from build123d import *

# Parameters (mm, degrees)
SKETCH046_R     = 1.5
PAD026_DEPTH    = 30
POCKET016_DEPTH = 19
POCKET017_DEPTH = 50
PAD027_DEPTH    = 3
PAD028_DEPTH    = 10
SKETCH054_W     = 30
SKETCH054_H     = 5.5
POCKET020_DEPTH = 9


with BuildPart() as part:
    # Sketch046 → Pad026 (new body)
    with BuildSketch(Plane.XY):
        with BuildLine():
            Line((-21.439893, 1.606546), (-18, 1))
            Line((-18, 1), (-18, 0))
            Line((-18, 0), (-20, 0))
            Line((-20, 0), (-20, -2))
            Line((-20, -2), (-18, -2))
            Line((-18, -2), (-18, -3))
            Line((-19.218253, -3.302841), (-18, -3))
            ThreePointArc((-19.218253, -3.302841), (-18.4595, -6.284654), (-17.241169, -9.11))
            Line((17.241169, -9.11), (-17.241169, -9.11))
            ThreePointArc((17.241169, -9.11), (18.417093, -6.407863), (19.172397, -3.559379))
            Line((19.172397, -3.559379), (16, -3))
            Line((16, -3), (16, -2))
            Line((16, -2), (18, -2))
            Line((18, -2), (18, 0))
            Line((18, 0), (16, 0))
            Line((16, 0), (16, 1))
            Line((16, 1), (21.411013, 1.954108))
            ThreePointArc((13, -17.124544), (19.673032, -8.673051), (21.411013, 1.954108))
            Line((13, -17.124544), (10, -17.124544))
            Line((10, -17.124544), (10, -10.124544))
            Line((10, -10.124544), (-10, -10.124544))
            Line((-10, -10.124544), (-10, -17.124544))
            Line((-10, -17.124544), (-13, -17.124544))
            ThreePointArc((-21.439893, 1.606546), (-19.60204, -8.832328), (-13, -17.124544))
        make_face()
        with Locations((-12.5, -15)):
            Circle(SKETCH046_R, mode=Mode.SUBTRACT)
        with Locations((12.5, -15)):
            Circle(SKETCH046_R, mode=Mode.SUBTRACT)
    extrude(amount=PAD026_DEPTH)

    # Sketch047 (on Face28 of Pad026) → Pocket016 (cut)
    with BuildSketch(Plane.XY.offset(30)):
        with BuildLine():
            ThreePointArc((-18.966908, -10.124544), (-16.362176, -13.947372), (-13, -17.124544))
            Line((-13, -17.124544), (13, -17.124544))
            ThreePointArc((13, -17.124544), (16.362176, -13.947372), (18.966908, -10.124544))
            Line((-18.966908, -10.124544), (18.966908, -10.124544))
        make_face()
    extrude(amount=-POCKET016_DEPTH, mode=Mode.SUBTRACT)

    # Sketch049 (on Face5 of Pocket016) → Pocket017 (cut)
    with BuildSketch(Plane.XY.offset(30)):
        with BuildLine():
            ThreePointArc((19.172397, -3.559379), (0, 19.5), (-19.172397, -3.559379))
            Line((19.172397, -3.559379), (-19.172397, -3.559379))
        make_face()
    extrude(amount=-POCKET017_DEPTH, mode=Mode.SUBTRACT)

    # Sketch048 (on Face5 of Pocket016) → Pad027 (join)
    with BuildSketch(Plane.XY.offset(30)):
        with BuildLine():
            ThreePointArc((-21.406775, 2), (-21.077469, -4.241496), (-18.966908, -10.124544))
            Line((-7.875644, -10.124544), (-18.966908, -10.124544))
            Line((-6, -17.124544), (-7.875644, -10.124544))
            Line((6, -17.124544), (-6, -17.124544))
            Line((6, -17.124544), (7.875644, -10.124544))
            Line((7.875644, -10.124544), (18.966908, -10.124544))
            ThreePointArc((18.966908, -10.124544), (20.278323, -7.144202), (21.12463, -4))
            Line((21.12463, -4), (22.264041, -3.25))
            ThreePointArc((22.264041, -3.25), (22.220442, 3.535811), (20.155644, 10))
            Line((15.730461, 10), (20.155644, 10))
            Line((12, 2), (15.730461, 10))
            Line((12, 2), (-21.406775, 2))
        make_face()
    extrude(amount=PAD027_DEPTH)

    # Sketch053 (on Face4 of Pad027) → Pad028 (join)
    with BuildSketch(Plane(origin=(0, 0, 30), x_dir=(1, 0, 0), z_dir=(0, 0, -1))):
        with BuildLine():
            ThreePointArc((20.155644, -10), (22.220442, -3.535811), (22.264041, 3.25))
            Line((22.264041, 3.25), (19.172397, 3.559379))
            ThreePointArc((16.740669, -10), (19.193782, -3.442198), (19.172397, 3.559379))
            Line((16.740669, -10), (20.155644, -10))
        make_face()
    extrude(amount=PAD028_DEPTH)

    # Sketch054 (on Face32 of Pad028) → Pocket020 (cut)
    with BuildSketch(Plane(origin=(0, 0, 20), x_dir=(1, 0, 0), z_dir=(0, 0, -1))):
        with Locations((15, -4.25)):
            Rectangle(SKETCH054_W, SKETCH054_H)
    extrude(amount=-POCKET020_DEPTH, mode=Mode.SUBTRACT)


with BuildPart() as part_1:
    # Body018 placement: moved
    add(part.part.moved(Location((0, 0, 200))))


solid = part_1.part
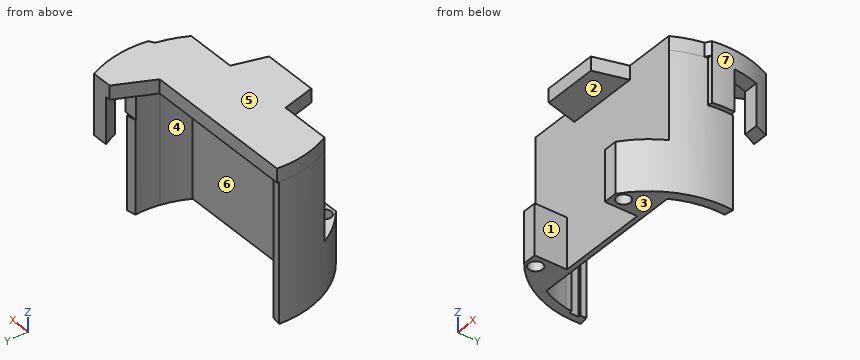
Part model, mm, in its own coordinate system. Face numbers are marked on the shaded views. A direction names the side the tool comes from. Coordinates: 2 decimals unless noted, no trailing zeros. Loops run counter-clockwise (first coordinate to the right, second up) from the corner with the lowest first, then second, coordinate; pieces in that order, holes last. Notation, with made-up numbers: M 89,7 L 96,7 A16 cw 96,18 Z; hole C 29.25,39 d5. An arc over 180 degrees is marked long. Use a Markdown table: item, result. Add a question column.
Q1. Cut at D-D (x = -5). Write the cut outline in (y, z), and give its area (3 significant figures).
Q2. Which spindle directions (+Z, -Z, +X, -X, +Y, -Y) get a long thin tool onto all of the face, cutting with end or side? Do the marked faces 1, 2, 3 and 4. Say none if no direction does.
Q3. Cut at A-A (z = 227). Write the cut outline in (x, y), and give its area (3 significant figures).
Q4. Probe L1, parallel to Y at x = -12.5, z = 204.75; L2, parallel to X at y = -16, z = 207.5; L3, parallel to X at y = -15, z = 208.75. List the from-to ranges inside material, lowest first.
Q5. Cut at C-C (z = 204). Write the cut outline in (x, y), and give its area (3 significant figures).
Q6. Mould opens along X. For the marked faces 5, 6 and 7 say: +X half, -X half, draft (parallel to the pull), parting line (faces both ways), or undercut.
Q7. Pin check, flat tips, straight feed: P1, Ø2, axis at y = -12, z = 207.5, coming from the -X side; P2, Ø2.5, axis at x = 19, y = 9, coming from the -Z side; P3, Ø1.5, axis at x = -8, z = 231, coming from the +Y side; P4, Ø2.5, axis at x = -12.5, y = -15, coming from the +Z side. Stop position of each tip, or through.
Q8. Cut at B-B (x = -12.5). Write the cut outline in (y, z).
Worked out:
| question | item | result |
|---|---|---|
| 1 | outline | M -17.12,230 L -10.12,230 L -10.12,200 L -9.11,200 L -9.11,230 L 2,230 L 2,233 L -17.12,233 Z |
| 1 | area | 87.8 mm2 |
| 2 | face 1 | +Z, -Z, -Y |
| 2 | face 2 | -Z, +X, -X, -Y |
| 2 | face 3 | -Z, +X, -X, +Y, -Y |
| 2 | face 4 | -Z |
| 3 | outline | M -21.44,1.61 A21.5 ccw -18.97,-10.12 L 18.97,-10.12 A21.5 ccw 21.24,-3.35 L 22.26,-3.25 A22.5 ccw 22.45,1.5 L 19.44,1.5 A19.5 cw 19.17,-3.56 A19.5 cw 17.24,-9.11 L -17.24,-9.11 A19.5 cw -19.22,-3.3 A19.5 cw -19.4,-2 L -20,-2 L -20,0 L -19.5,0 A19.5 cw -19.46,1.26 Z; M 16.74,10 A19.5 cw 18.2,7 L 21.38,7 A22.5 ccw 20.16,10 Z |
| 3 | area | 96.3 mm2 |
| 4 | L1 | y = -17.12 to -16.5, -13.5 to -9.11 |
| 4 | L2 | x = -14.36 to -13.62, -11.38 to -10, 10 to 11.38, 13.62 to 14.36 |
| 4 | L3 | x = -15.4 to -14, -11 to -10, 10 to 11, 14 to 15.4 |
| 5 | outline | M -21.44,1.61 A21.5 ccw -13,-17.12 L -10,-17.12 L -10,-10.12 L 10,-10.12 L 10,-17.12 L 13,-17.12 A21.5 ccw 21.41,1.95 L 19.43,1.61 A19.5 cw 19.17,-3.56 A19.5 cw 17.24,-9.11 L -17.24,-9.11 A19.5 cw -19.22,-3.3 A19.5 cw -19.4,-2 L -20,-2 L -20,0 L -19.5,0 A19.5 cw -19.46,1.26 Z; hole C -12.5,-15 d3; hole C 12.5,-15 d3 |
| 5 | area | 158 mm2 |
| 6 | face 5 | draft |
| 6 | face 6 | undercut |
| 6 | face 7 | +X half |
| 7 | P1 | stops at x = -18.47 |
| 7 | P2 | stops at z = 220 |
| 7 | P3 | stops at y = 2 |
| 7 | P4 | passes through |
| 8 | outline | M -17.12,200 L -16.5,200 L -16.5,211 L -17.12,211 Z; M -13.5,200 L -9.11,200 L -9.11,230 L 2,230 L 2,233 L -10.12,233 L -10.12,211 L -13.5,211 Z |
